Input: part model. Units: mm. Frame: model coordinates. Face numbers are marked on the shaded views. A direction names the side the tool comes from. Coordinates: 2 decimals unless noted, no trailing zeros. Write each loop counter-clockwise with the first axis right and the second up, starting at its lowest first coordinate (ties: lowest second). Pieces come first, ordered by that corner, then holes. Notation, with made-up numbers: (-33, 43.5) -> (-27, 43.5) arc R22 cw to (-27, 69.5) -> close; hole circle Ø11 at (12.5, 67). An arc over 180 degrees is marked (long way). Use one line per item in the form item = value. Start each with the question number.
(1) First-contact query: pin 1 (0.9 mm diameter, centred on y = 5, z = -17.5, fed in from -X); pin 2 (2.5 mm diameter, centred on x = -7.03, y = 4.25, fed in from +Z). Flat tips, straight axial feed; report the tip coordinate or a pass-through.
(2) Cut plane B-B on z = -12. Return the cut outline in (x, y).
(3) Cut plane A-A on x = 7. Return the cut outline in (y, z).
(4) Set-up query: the marked faces 1, 2 and 3. Return all of +Z, -Z, +X, -X, +Y, -Y with unobstructed straight access to the full face (end or side cutting, diameter ignored); none if empty.
(5) Cut plane D-D on y = 7.75. Return the cut outline in (x, z), plus the area to 3 significant figures.
(6) Cut plane C-C on z = -2. Return the cut outline in (x, y).
(7) Pull-direction query (Y, two-part tool) for the marked faces 4, 5 and 6; classes: released by +Y, released by -Y, zero draft, split by the parting line, or undercut.
(8) Ray query, line 1 along Z through (x, y) = (6.75, 5.75); line 2 along X through (y, z) = (6.5, -16.5); line 3 along X through (y, z) = (2, -5.5). Return the intervals inside material, ascending.
```python
from build123d import *

# Parameters (mm, degrees)
BOSS_EXTRUDE1_DEPTH                                 = 8.5
CUT_EXTRUDE1_REACH                                  = 35.245
SKETCH2_R                                           = 1.5
FILLET1_R                                           = 5
FILLET2_R                                           = 2
CSK_FOR_M3_COUNTERSUNK_FLAT_HEAD_SCREW1_D           = 3.4
CSK_FOR_M3_COUNTERSUNK_FLAT_HEAD_SCREW1_CSINK_D     = 6.3
CSK_FOR_M3_COUNTERSUNK_FLAT_HEAD_SCREW1_CSINK_ANGLE = 90
CUT_EXTRUDE2_DEPTH                                  = 3


with BuildPart() as part:
    # Sketch1 → Boss-Extrude1 (new body)
    with BuildSketch(Plane(origin=(0, 0, 0), x_dir=(1, 0, 0), z_dir=(0, 1, 0))):
        Polygon((-11.531971071, 19.053328449), (9.218028929, 19.053328449), (9.218028929, 11.553328449), (4.218028929, 11.553328449), (4.218028929, -3.446671551), (9.218028929, -3.446671551), (9.218028929, -10.946671551), (-11.531971071, -10.946671551), (-11.531971071, -3.446671551), (-1.531971071, -3.446671551), (-1.531971071, 11.553328449), (-11.531971071, 11.553328449), align=None)
    extrude(amount=BOSS_EXTRUDE1_DEPTH)

    # Cut-Extrude1: up to this face of the body (flat: up to its plane)
    cut_extrude1_end = Plane(part.part.faces().sort_by_distance((-1.156971071, 4.25, -19.053328449))[0])
    # Sketch2 → Cut-Extrude1 (cut, up to the picked face)
    with BuildSketch(Plane.XY.offset(10.946671551), mode=Mode.PRIVATE) as cut_extrude1_sk1:
        with Locations((-7.031971071, 4.25)):
            Circle(SKETCH2_R)
    cut_extrude1_tool1 = split(extrude(cut_extrude1_sk1.sketch, amount=-CUT_EXTRUDE1_REACH, mode=Mode.PRIVATE), bisect_by=cut_extrude1_end, keep=Keep.BOTH, mode=Mode.PRIVATE)
    add(cut_extrude1_tool1.solids().sort_by(Axis((-7.031971, 4.25, 10.946672), (0, 0, -1)))[0], mode=Mode.SUBTRACT)

    # Fillet1
    # the kernel refuses this fillet: 5 mm, written as the material it takes off along each edge
    with BuildSketch(Plane(origin=(-11.531971071, 0, 0.946671551), x_dir=(0, 1, 0), z_dir=(0, 0, -1)), Plane(origin=(-11.531971071, 8.5, 23.446671551), x_dir=(1, 0, 0), z_dir=(0, 0, -1))) as fillet1_piece_1:
        with BuildLine():
            CenterArc((FILLET1_R, FILLET1_R), FILLET1_R, 180, 90)
            Line((0, FILLET1_R), (0, 0))
            Line((0, 0), (FILLET1_R, 0))
        make_face()
    extrude(amount=32.5, mode=Mode.SUBTRACT)
    with BuildSketch(Plane(origin=(-11.531971071, 8.5, 0.946671551), x_dir=(0, -1, 0), z_dir=(0, 0, -1)), Plane(origin=(-11.531971071, 0, 23.446671551), x_dir=(1, 0, 0), z_dir=(0, 0, -1))) as fillet1_piece_2:
        with BuildLine():
            CenterArc((FILLET1_R, -FILLET1_R), FILLET1_R, 90, 90)
            Line((0, -FILLET1_R), (0, 0))
            Line((0, 0), (FILLET1_R, 0))
        make_face()
    extrude(amount=32.5, mode=Mode.SUBTRACT)

    # Fillet2
    # the kernel refuses this fillet: 2 mm, written as the material it takes off along each edge
    with BuildSketch(Plane(origin=(-11.531971071, 0, -19.053328449), x_dir=(0, 1, 0), z_dir=(1, 0, 0)), Plane(origin=(14.218028929, 8.5, 10.946671551), x_dir=(0, 0, -1), z_dir=(-1, 0, 0))) as fillet2_piece_1:
        with BuildLine():
            CenterArc((FILLET2_R, FILLET2_R), FILLET2_R, 180, 90)
            Line((0, FILLET2_R), (0, 0))
            Line((0, 0), (FILLET2_R, 0))
        make_face()
    extrude(amount=25.75, mode=Mode.SUBTRACT)
    with BuildSketch(Plane(origin=(-11.531971071, 8.5, -19.053328449), x_dir=(0, -1, 0), z_dir=(1, 0, 0)), Plane(origin=(14.218028929, 0, 10.946671551), x_dir=(0, 0, -1), z_dir=(-1, 0, 0))) as fillet2_piece_2:
        with BuildLine():
            CenterArc((FILLET2_R, -FILLET2_R), FILLET2_R, 90, 90)
            Line((0, -FILLET2_R), (0, 0))
            Line((0, 0), (FILLET2_R, 0))
        make_face()
    extrude(amount=25.75, mode=Mode.SUBTRACT)

    # CSK for M3 Countersunk Flat Head Screw1 (through all)
    with Locations(Plane.XY.offset(10.946671551)):
        with Locations((-7.031971071, 4.25)):
            CounterSinkHole(CSK_FOR_M3_COUNTERSUNK_FLAT_HEAD_SCREW1_D / 2, CSK_FOR_M3_COUNTERSUNK_FLAT_HEAD_SCREW1_CSINK_D / 2, counter_sink_angle=CSK_FOR_M3_COUNTERSUNK_FLAT_HEAD_SCREW1_CSINK_ANGLE)

    # Sketch5 → Cut-Extrude2 (cut)
    with BuildSketch(Plane(origin=(0, 0, -19.053328449), x_dir=(-1, 0, 0), z_dir=(0, 0, -1))):
        Polygon((7.031971071, 7.425426481), (4.281971071, 5.83771324), (4.281971071, 2.66228676), (7.031971071, 1.074573519), (9.781971071, 2.66228676), (9.781971071, 5.83771324), align=None)
    extrude(amount=-CUT_EXTRUDE2_DEPTH, mode=Mode.SUBTRACT)


solid = part.part
```
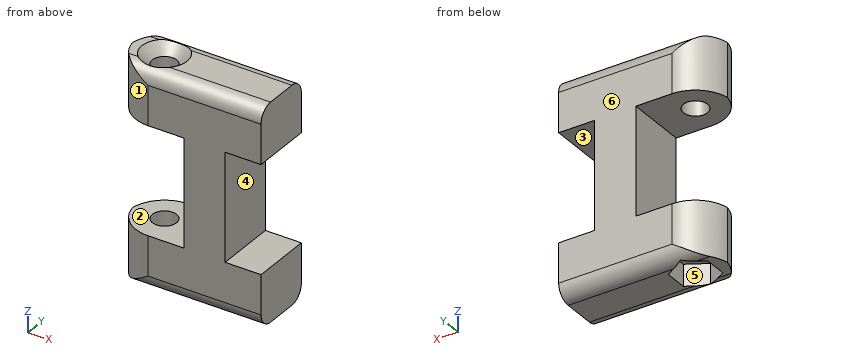
Values:
q1.pin_1 = -11.42
q1.pin_2 = through
q2.outline = (-11.48, 4.25) arc R5 ccw to (-6.53, 0) -> (9.22, 0) -> (9.22, 8.5) -> (-6.53, 8.5) arc R5 ccw to start; hole circle Ø3.4 at (-7.03, 4.25)
q3.outline = (0, -17.05) arc R2 ccw to (2, -19.05) -> (6.5, -19.05) arc R2 ccw to (8.5, -17.05) -> (8.5, -11.55) -> (0, -11.55) -> close; (0, 3.45) -> (8.5, 3.45) -> (8.5, 8.95) arc R2 ccw to (6.5, 10.95) -> (2, 10.95) arc R2 ccw to (0, 8.95) -> close
q4.face_1 = +Z, -Z, -X, -Y
q4.face_2 = -X, +Y, -Y
q4.face_3 = +X, +Y, -Y
q5.outline = (-9.17, -18.61) -> (9.22, -18.61) -> (9.22, -11.55) -> (4.22, -11.55) -> (4.22, 3.45) -> (9.22, 3.45) -> (9.22, 10.51) -> (-9.17, 10.51) -> (-9.17, 3.45) -> (-1.53, 3.45) -> (-1.53, -11.55) -> (-9.17, -11.55) -> close
q5.area = 346 mm2
q6.outline = (-1.53, 0) -> (4.22, 0) -> (4.22, 8.5) -> (-1.53, 8.5) -> close
q7.face_4 = zero draft
q7.face_5 = undercut
q7.face_6 = released by +Y
q8.line_1 = -19.05 to -11.55, 3.45 to 10.95
q8.line_2 = -10.53 to -8.63, -5.43 to 9.22
q8.line_3 = -1.53 to 4.22
